Geometry: final body of the model. Coordinates: model frame, mm. Round coordinates to 2 decimals unless told otherwise and drop trailing zeros. Write each loop counter-clockwise with the first axis right and the second up, starting at its lowest first coordinate (ties: lowest second). Pieces come first, ordered by that corner, then holes. Notation, with made-up numbers: M -17.75,-31.5 L 17.25,-31.5 A7 ccw 17.25,-25.5 Z; hole C 45.5,61 d5. An arc over 180 degrees is marked long. Use one line per item in the form item = value. Start each with the question number.
Item 1: Section query C-C (x = 453.5). Return loops of the section in (y, z), and give its area (3 significant figures).
Item 2: Pin query (flat end, axial travel): pin 1 Ø5.5 at (y, z) = (0, 0) entering from -X; pin 2 Ø3 at (x, y) = (291.5, -5) entering from -Z; pin 3 Ø1 at (y, z) = (-3.5, 3) entering from -X. Return the tip coordinate at first contact, or that it passes through.
Item 3: Ray query, probe 1 along Y at (x, z) = (0.15, 0) (3 decimals); probe 2 along X at (y, z) = (-2, 3.5); probe 3 along X at (y, z) = (-1.25, -2.25). Return the intervals inside material, ascending.
from build123d import *

# Parameters (mm, degrees)
FILLET1_R           = 0.4
SKETCH6_R           = 5.25
BOSS_EXTRUDE1_DEPTH = 853.2
SKETCH7_R           = 3.175
CUT_EXTRUDE1_DEPTH  = 0.2
SKETCH9_R           = 3.175
CUT_EXTRUDE2_DEPTH  = 0.2


with BuildPart() as part:
    # Sketch3 → Revolve1 (revolve)
    with BuildSketch(Plane.XY, mode=Mode.PRIVATE) as revolve1_sk:
        Polygon((0, 0), (0, 3.95), (13.1, 3.95), (13.1, 6.05), (28.4, 6.05), (28.4, 0), align=None)
    revolve1 = revolve(revolve1_sk.sketch.rotate(Axis((0, 0, 0), (1, 0, 0)), 90), axis=Axis((0, 0, 0), (1, 0, 0)))  # turned: the seam where the file's is

    # Fillet1
    fillet1_edges = [part.edges().sort_by_distance(p)[0] for p in [
        (13.1, 0, -3.95),
    ]]
    fillet(fillet1_edges, radius=FILLET1_R)

    # Sketch6 → Boss-Extrude1 (add)
    with BuildSketch(Plane(origin=(28.4, 0, 0), x_dir=(0, 0, -1), z_dir=(1, 0, 0))):
        with Locations(Location((0, 0, 0), (0, 0, 180))):  # turned: the seam where the file's is
            Circle(SKETCH6_R)
    extrude(amount=BOSS_EXTRUDE1_DEPTH)

    # Mirror1: Revolve1 across plane
    add(revolve1.mirror(Plane(origin=(455, 0, 0), x_dir=(0, 0, 1), z_dir=(1, 0, 0))))

    # Sketch7 → Cut-Extrude1 (cut)
    with BuildSketch(Plane(origin=(910, 0, 0), x_dir=(0, 0, -1), z_dir=(1, 0, 0))):
        Circle(SKETCH7_R)
    extrude(amount=-CUT_EXTRUDE1_DEPTH, mode=Mode.SUBTRACT)

    # Sketch9 → Cut-Extrude2 (cut)
    with BuildSketch(Plane.ZY):
        with Locations(Location((0, 0, 0), (0, 0, 180))):  # turned: the seam where the file's is
            Circle(SKETCH9_R)
    extrude(amount=-CUT_EXTRUDE2_DEPTH, mode=Mode.SUBTRACT)


solid = part.part
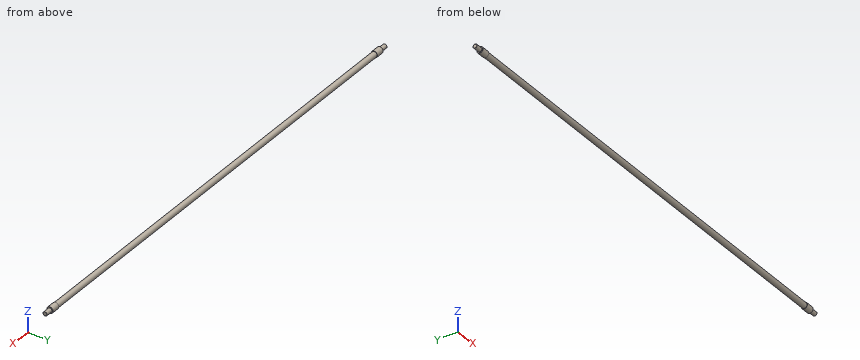
Working result:
q1.outline = C 0,0 d10.5
q1.area = 86.6 mm²
q2.pin_1 = 0.2
q2.pin_2 = -3.91
q2.pin_3 = 13.02
q3.probe_1 = -3.95 to -3.175, 3.175 to 3.95
q3.probe_2 = 12.94 to 896.9
q3.probe_3 = 0.2 to 909.8
